For this review, take the finished solid that the model builds, in its own axes (mm). Face numbers are marked on the shaded views. A direction names the side the tool comes from. Give positions to 0.01 mm unless a question says otherwise; leave off trailing zeros. Loops run counter-clockwise (first coordinate to the right, second up) from the corner with the lowest first, then second, coordinate; pieces in that order, holes last.
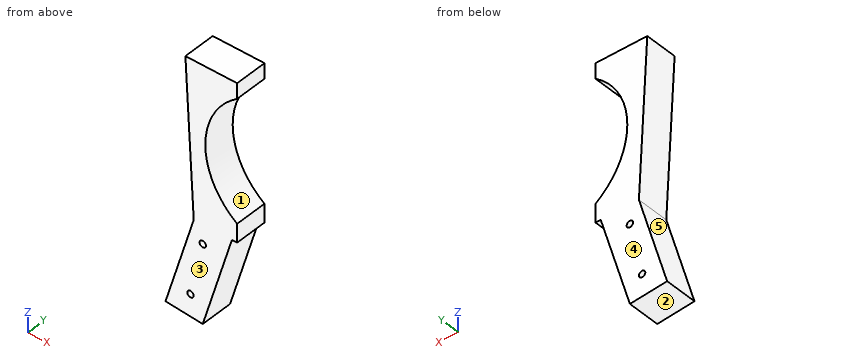
```python
from build123d import *

# Parameters (mm, degrees)
F0_R     = 1.5571839485
F0_R_2   = 1.582453361
F1_DEPTH = 7.9375


# Not quite as in the source:
# - a feature names something its author has since deleted; it is built from what else it names


with BuildPart() as f1:
    # F0 (on Front) → F1 (new body, symmetric)
    with BuildSketch(Plane.XZ):
        with BuildLine():
            Line((-4.4244504534, -9.0134367347), (14.3148868547, -9.0134367347))
            Line((14.3148868547, -9.0134367347), (16.876486437, -9.0134367347))
            Line((16.876486437, -9.0134367347), (16.876486437, 0))
            ThreePointArc((16.876486437, 0), (1.2674691421, 29.8639013079), (16.876486437, 59.7278026158))
            Line((16.876486437, 59.7278026158), (16.876486437, 67.1865632653))
            Line((16.876486437, 67.1865632653), (-8.523513563, 67.1865632653))
            Line((-8.523513563, 67.1865632653), (-4.4244504534, -9.0134367347))
        make_face()
        Polygon((0, -56.506741792), (14.3148868547, -9.0134367347), (-4.4244504534, -9.0134367347), (-18.2776516019, -54.9749811636), align=None)
        with Locations((-6.0080750845, -45.2978610992)):
            Circle(F0_R, mode=Mode.SUBTRACT)
        with Locations((0, -18.3103610992)):
            Circle(F0_R_2, mode=Mode.SUBTRACT)
    extrude(amount=F1_DEPTH, both=True)


solid = f1.part
```
Q1. Consider section C-C on z = 6.5. Give the boundary of the cut face in (x, y), plus the area to 3 significant figures.
Answers:
outline: (-5.26, -7.94) - (9.76, -7.94) - (9.76, 7.94) - (-5.26, 7.94) - close
area: 238 mm2
Q2. Consider section A-A on x = 5.5. Give the boundary of the cut face in (y, z), plus the area to 3 significant figures.
Answers:
outline: (-7.94, -38.26) - (7.94, -38.26) - (7.94, 12.83) - (-7.94, 12.83) - close; (-7.94, 46.89) - (7.94, 46.89) - (7.94, 67.19) - (-7.94, 67.19) - close
area: 1,130 mm2
Q3. Mouldability with a two-part tool opening along Z and no side actions: class the marked faces 1, 2 and 3 as +Z half, -Z half, draft (parallel to the pull), parting line (faces both ways), or undercut.
Answers:
face 1: undercut
face 2: -Z half
face 3: draft
Q4. Machinability: for the marked faces 4 and 5, which of the approach directions +Z, -Z, +X, -X, +Y, -Y give a long, thin tool a straight path to every point of the face, cutting with its end or side? Answer none if there is none.
Answers:
face 4: +Z, -Z, +X, -X, +Y
face 5: -X, +Y, -Y
Q5. Consider section B-B on y = 6. Give the boundary of the cut face in (x, z).
Answers:
outline: (-18.28, -54.97) - (0, -56.51) - (14.31, -9.01) - (16.88, -9.01) - (16.88, 0) arc R36.37 cw to (16.88, 59.73) - (16.88, 67.19) - (-8.52, 67.19) - (-4.42, -9.01) - close; hole circle Ø3.11 at (-6.01, -45.3); hole circle Ø3.16 at (0, -18.31)
Q6. Consider section D-D on x = -11. Give the boundary of the cut face in (y, z).
Answers:
outline: (-7.94, -55.58) - (7.94, -55.58) - (7.94, -30.83) - (-7.94, -30.83) - close
Q7. For probe 1 along Z at (x, y) = (14.5, 3); probe 2 along X at (y, z) = (5.5, 57.5); probe 3 along X at (y, z) = (-7, 5), list the stretches that pass through material, from the lowest coordinate up.
Answers:
probe 1: z = -9.01 to 1.8, 57.93 to 67.19
probe 2: x = -8 to 13.99
probe 3: x = -5.18 to 11.09
Q8. For pin 1 Ø5 at (x, y) = (-9, -2.5) entering from -Z; pin 2 Ø2 at (y, z) = (0.5, -12) entering from -X; pin 3 Ø6 at (y, z) = (4.5, -33.5) entering from +X, all flat-tipped, find the tip position at first contact; note any pin that passes through.
Answers:
pin 1: stops at z = -55.96
pin 2: stops at x = -5.63
pin 3: stops at x = 7.84
